The listing builds one solid part. Answer for the finished solid, in the listing's coordinates (mm). A direction names the side the tool comes from. Give positions to 0.01 mm unless a question says otherwise; leave off trailing zeros. Write each loop counter-clockwise with the first axis right and the second up, starting at its lowest first coordinate (ties: lowest second). Pieces come first, ordered by that corner, then holes. Notation, with made-up numbers: (77, 19.25) - (107, 19.25) arc R29 cw to (107, 58.25) - close; hole circle Ø8 at (63.25, 1.5). An arc over 180 degrees is marked (long way). Return JSON: item names as keys, results as strings.
from build123d import *

# Parameters (mm, degrees)
CHAMFER_1_SIZE = 0.5
CHAMFER_2_SIZE = 0.1


with BuildPart() as part:
    # ｽｹｯﾁ1 → 回転1 (revolve)
    with BuildSketch(Plane.XY, mode=Mode.PRIVATE) as revolve_1_sk:
        Polygon((43.5, 4), (-43.5, 4), (-43.5, 3), (-51.5, 3), (-51.5, 0), (51.5, 0), (51.5, 3), (43.5, 3), align=None)
    revolve(revolve_1_sk.sketch.rotate(Axis((-61.290700214, 0, 0), (1, 0, 0)), 90), axis=Axis((-61.290700214, 0, 0), (1, 0, 0)))

    # 面取り1
    chamfer_1_edges = [part.edges().sort_by_distance(p)[0] for p in [
        (-51.5, 0, -3),
        (51.5, 0, -3),
    ]]
    chamfer(chamfer_1_edges, length=CHAMFER_1_SIZE)

    # 面取り2
    chamfer_2_edges = [part.edges().sort_by_distance(p)[0] for p in [
        (-43.5, 0, -4),
        (43.5, 0, -4),
    ]]
    chamfer(chamfer_2_edges, length=CHAMFER_2_SIZE)

    # ｽｹｯﾁ3 → M3 ねじ穴1 (revolve, cut)
    with BuildSketch(Plane(origin=(51.5, 0, 0), x_dir=(0, 0, -1), z_dir=(0, 1, 0))):
        Polygon((0, 0), (0, 9.251075774), (1.25, 8.5), (1.25, 0), align=None)
    hole_wizard_m3_1 = revolve(axis=Axis((57.85, 0, 0), (-1, 0, 0)), mode=Mode.SUBTRACT)

    # ﾐﾗｰ1: M3 ねじ穴1 across plane
    add(hole_wizard_m3_1.mirror(Plane(origin=(0, 0, 0), x_dir=(0, 0, 1), z_dir=(1, 0, 0))), mode=Mode.SUBTRACT)


solid = part.part
Item 1: The mould has two halves that part along Y. Classify faces 4 (the face through (-0.608, 3.905, -0.867)), 5 (the face through (51.5, -1, -1)), 6 (the face through (-42.38, 0.21, 0.05)): +Y half, -Y half, draft (parallel to the pull), parting line (faces both ways), or undercut.
Answer below:
{"face 4": "parting line", "face 5": "draft", "face 6": "undercut"}
Item 2: Consider L1, parallel to Y at x = -49.25, z = 0; L2, parallel to X at y = 3.75, z = -0.5; L3, parallel to Z at x = -35, y = 0.25. Determine where each line is inside the solid, lowest interval first.
Answer below:
{"L1": "y = -3 to -1.25, 1.25 to 3", "L2": "x = -43.5 to 43.5", "L3": "z = -3.99 to 3.99"}
Item 3: A cutting plane is placed at A-A on x = -6. Determine the outline of the cut face in (y, z).
Answer below:
{"outline": "circle Ø8 at (0, 0)"}
Item 4: For faces 1 (the face through (-51.5, -1, 1)), 2 (the face through (-47.3, -0.9, 2.86)), 3 (the face through (47.2, -0.9, 2.86)), determine the directions among +Z, -Z, +X, -X, +Y, -Y from which every point of the face is accessible in a straight line to the end or side of a thin tool.
Answer below:
{"face 1": "+Z, -Z, -X, +Y, -Y", "face 2": "-X", "face 3": "+X"}
Item 5: A flat-ended cylindrical pin translates along its axis: P1, Ø2, axis at y = 0, z = 0, coming from the -X side. Find the tip coordinate at first contact, or state that the pin passes through.
Answer below:
{"P1": "stops at x = -42.85"}
